Autodesk Inventor part; units mm, degrees
ref_plane "YZ Plane" through (0, 0, 0) normal (1, 0, 0) x (0, 1, 0)
ref_plane "XZ Plane" through (0, 0, 0) normal (0, 1, 0) x (-1, 0, 0)
ref_plane "XY Plane" through (0, 0, 0) normal (0, 0, 1) x (1, 0, 0)
sketch "Skizze1" plane through (0, 0, 0) normal (0, 1, 0) x (-1, 0, 0)
  line L0 (45.2756, -27.3622) -> (15.2756, -27.3622)
  line L1 (15.2756, -27.3622) -> (15.2756, -77.3622)
  line L2 (15.2756, -77.3622) -> (45.2756, -77.3622)
  line L3 (45.2756, -77.3622) -> (45.2756, -27.3622)
  point P0 (0, 0)
  dimension "d0" = 50
  dimension "d1" = 30
extrude "Extrusion1" add sketch "Skizze1" along normal blind 3
sketch "Skizze2" plane through (0, 3, 0) normal (0, 1, 0) x (1, 0, 0)
  circle A0 centre (-30.2756, 39.3622) radius 10
  circle A1 centre (-30.2756, 65.3622) radius 10
  line L0 (-45.2756, 77.3622) -> (-45.2756, 27.3622)
  line L1 (-45.2756, 27.3622) -> (-15.2756, 27.3622)
  line L2 (-15.2756, 77.3622) -> (-45.2756, 77.3622)
  point P0 (0, 0)
  dimension "d4" = 20
  dimension "d5" = 20
  dimension "d6" = 15
  dimension "d7" = 15
  dimension "d10" = 12
  dimension "d11" = 12
extrude "Extrusion2" add sketch "Skizze2" along normal blind 15
properties part number "Ultraschallsensor"
CAD build for the part. Positions are in the model's coordinates, mm. A direction names the side the tool comes from. Give positions to 0.01 mm unless a question says otherwise; leave off trailing zeros. Order: outer loops, then holes, each group sorted by start corner. A loop starts at its lowest first (then second) coordinate and runs counter-clockwise, first axis right, second up. Notation, with made-up numbers: (-9, 11) - (30, 11) arc R33 ccw to (30, 47) - close; hole circle Ø9 at (84, 43.25). An arc over 180 degrees is marked (long way). Answer in a Markdown table with one row per item.
1. Saw through at A-A, the plane x = -32.5. Give the cut face in (y, z).
Data:
| item | result |
|---|---|
| outline | (0, -77.36) - (3, -77.36) - (3, -75.11) - (18, -75.11) - (18, -55.61) - (3, -55.61) - (3, -49.11) - (18, -49.11) - (18, -29.61) - (3, -29.61) - (3, -27.36) - (0, -27.36) - close |
2. Flat gauge pins, fed straight in: pin 1 (10 mm diameter, centred on x = -39, y = 9.5, fed in from +Z); pin 2 (2 mm diameter, centred on y = 12.5, z = -51.5, fed in from -X); pin 3 (4 mm diameter, centred on y = 14.5, z = -37.5, fed in from -X). Where does each tip first touch, or does it go through?
Data:
| item | result |
|---|---|
| pin 1 | stops at z = -30.08 |
| pin 2 | passes through |
| pin 3 | stops at x = -40.28 |
3. Probe probe 1 along Y at (x, z) = (-17.75, -64); probe 2 along Z at (x, y) = (-38.25, 5.5); probe 3 along Z at (x, y) = (-37.75, 16.25). List the from-to ranges inside material, lowest first. Write a range as [from, to].
Data:
| item | result |
|---|---|
| probe 1 | y = [0, 3] |
| probe 2 | z = [-71.4, -59.33], [-45.4, -33.33] |
| probe 3 | z = [-72.01, -58.72], [-46.01, -32.72] |
4. Saw through at D-D, the plane x = -38.5. Give the cut face in (y, z).
Data:
| item | result |
|---|---|
| outline | (0, -77.36) - (3, -77.36) - (3, -71.05) - (18, -71.05) - (18, -59.67) - (3, -59.67) - (3, -45.05) - (18, -45.05) - (18, -33.67) - (3, -33.67) - (3, -27.36) - (0, -27.36) - close |
5. Saw through at C-C, the plane y = 13.25. Give the cut face in (x, z), plus the area to 3 significant figures.
Data:
| item | result |
|---|---|
| outline | circle Ø20 at (-30.28, -65.36); circle Ø20 at (-30.28, -39.36) |
| area | 628 mm² |
6. Saw through at B-B, the plane z = -42.5. Give the cut face in (x, y).
Data:
| item | result |
|---|---|
| outline | (-45.28, 0) - (-15.28, 0) - (-15.28, 3) - (-20.78, 3) - (-20.78, 18) - (-39.77, 18) - (-39.77, 3) - (-45.28, 3) - close |
7. Pull direction Z, two halves, no side cores. Call faces 1 (the flat face through (-30, 3, -52)), 2 (the flat face through (-30, 18, -40)), 3 (the flat face through (-30, 1, -77.362)): pulls with the +Z half, pulls with the -Z half, needs draft (parallel to the pull), parting line crosses it, or undercut.
Data:
| item | result |
|---|---|
| face 1 | undercut |
| face 2 | needs draft |
| face 3 | pulls with the -Z half |
8. Tool access for faces 4 (the cylindrical face through (-21.038, 10.395, -43.192)), 5 (the flat face through (-30, 18, -66)): list every direction of +Z, -Z, +X, -X, +Y, -Y with a clear straight run to the whole face (end or side of a thin tool).
Data:
| item | result |
|---|---|
| face 4 | +Y |
| face 5 | +Z, -Z, +X, -X, +Y |
